Verification items for the finished model (mm, model axes). Coordinates: 2 decimals unless noted, no trailing zeros. Order: outer loops, then holes, each group sorted by start corner. A loop starts at its lowest first (then second) coordinate and runs counter-clockwise, first axis right, second up.
Q1. Cross-section at C-C, the plane x = 60.5. Record the boundary of the cut face in (y, z) (3 decimals).
Q2. Draft check along Y on faces 1 (the flat face through (38, 9.525, 1)), 2 (the flat face through (66.675, 25, 1)), 3 (the cylindrical face through (62.683, 13.596, 0.986)), 4 (the cylindrical face through (16.38, 13.6, 0.99)). Enter one of: pulls with the +Y half, pulls with the -Y half, needs draft (parallel to the pull), parting line crosses it, or undercut.
Q3. Cross-section at A-A, the plane x = 15. Record the boundary of the cut face in (y, z) (3 decimals).
Q4. Thickness scan on line 1 (X direction, y = 14, z = 1.35) (3 decimals). Record the ranges inside material, lowest first.
Q5. Cross-section at B-B, the plane z = 0.4. Record the boundary of the cut face in (x, y) (3 decimals), and give its area (3 significant figures).
Autodesk Inventor part; units mm, degrees
ref_plane "YZ Plane" through (0, 0, 0) normal (1, 0, 0) x (0, 1, 0)
ref_plane "XZ Plane" through (0, 0, 0) normal (0, 1, 0) x (-1, 0, 0)
ref_plane "XY Plane" through (0, 0, 0) normal (0, 0, 1) x (1, 0, 0)
sketch "Sketch1" plane through (0, 0, 0) normal (0, 0, 1) x (1, 0, 0)
  line L0 (0, 0) -> (0, 50.8)
  line L1 (0, 50.8) -> (76.2, 50.8)
  line L2 (76.2, 50.8) -> (76.2, 0)
  line L3 (76.2, 0) -> (0, 0)
  circle A0 centre (61.2521, 14.0462) radius 1.5
  circle A1 centre (14.9479, 14.0462) radius 1.5
  circle A2 centre (61.2521, 36.7538) radius 1.5
  circle A3 centre (14.9479, 36.7538) radius 1.5
  line L4 (14.9479, 36.7538) -> (14.9479, 14.0462)
  line L5 (0, 25.4) -> (-9.2458, 25.4)
  line L6 (66.675, 41.275) -> (9.525, 41.275)
  line L7 (9.525, 41.275) -> (9.525, 9.525)
  line L8 (9.525, 9.525) -> (66.675, 9.525)
  line L9 (66.675, 9.525) -> (66.675, 41.275)
  dimension "d0" = 50.8
  dimension "d1" = 76.2
  dimension "d2" = 3
  dimension "d3" = 3
  dimension "d4" = 9.525
extrude "Extrusion1" add sketch "Sketch1" along normal blind 2 contours L9 L8 L7 L6
properties part number "baseplate"
Check values:
1. outline: (9.525, 0) - (12.748, 0) - (12.748, 2) - (9.525, 2) - close; (15.344, 0) - (35.456, 0) - (35.456, 2) - (15.344, 2) - close; (38.052, 0) - (41.275, 0) - (41.275, 2) - (38.052, 2) - close
2. face 1: pulls with the -Y half
2. face 2: needs draft
2. face 3: undercut
2. face 4: undercut
3. outline: (9.525, 0) - (12.547, 0) - (12.547, 2) - (9.525, 2) - close; (15.545, 0) - (35.255, 0) - (35.255, 2) - (15.545, 2) - close; (38.253, 0) - (41.275, 0) - (41.275, 2) - (38.253, 2) - close
4. line 1: x = 9.525 to 13.449, 16.447 to 59.753, 62.751 to 66.675
5. outline: (9.525, 9.525) - (66.675, 9.525) - (66.675, 41.275) - (9.525, 41.275) - close; hole circle Ø3 at (14.948, 14.046); hole circle Ø3 at (14.948, 36.754); hole circle Ø3 at (61.252, 14.046); hole circle Ø3 at (61.252, 36.754)
5. area: 1,790 mm2
